Verification items for this drawing (mm, ordinates from the low corner). A direction names the side the tool comes from. Give positions to 0.01 mm unless a question says otherwise; leave off trailing zeros. Write each loop counter-clockwise with the first axis right and the second up, starting at its lowest first coordinate (ties: lowest second). Pieces come first, ordered by that corner, then holes. Notation, with made-up numbers: (8.25, -5.75) -> (47.25, -5.75) arc R28 ccw to (47.25, 30.25) -> close; hole circle Ø9 at (5, 45.5). An arc over 180 degrees is marked (long way). Answer as a JSON object with one key per item and string values.
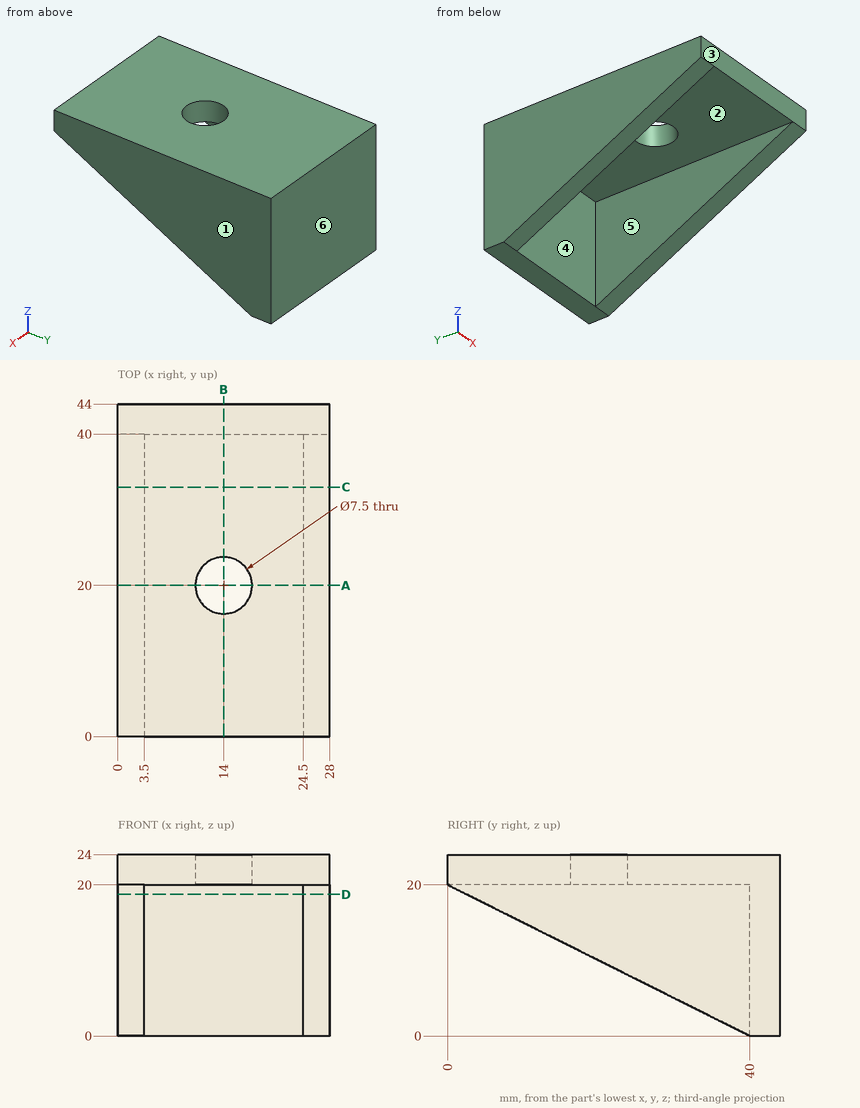
1. Sectioned sample at C-C, the plane y = 33. Enter the section's corners in (x, z), plus the area to 4 significant figures.
Determined:
{"outline": "(0, 3.5) -> (3.5, 3.5) -> (3.5, 20) -> (24.5, 20) -> (24.5, 3.5) -> (28, 3.5) -> (28, 24) -> (0, 24) -> close", "area": "227.5 mm^2"}
2. Scan lines: L1, parallel to Y at x = 14, z = 22.6; L2, parallel to X at y = 34, z = 13.5; L3, parallel to Z at x = 18.5, y = 37. Record each from-to range of solid material in increasing order. Write a range as [from, to].
Determined:
{"L1": "[0, 16.25], [23.75, 44]", "L2": "[0, 3.5], [24.5, 28]", "L3": "[20, 24]"}
3. Mould release check, pull along X, two halves, no side actions. Record for the marked faces 1, 2, 3 and 4: released by +X, released by -X, zero draft, split by the parting line, or undercut.
Determined:
{"face 1": "released by +X", "face 2": "undercut", "face 3": "zero draft", "face 4": "undercut"}
4. Sectioned sample at B-B, the plane x = 14. Enter the section's corners in (y, z), plus the area to 3 significant figures.
Determined:
{"outline": "(0, 20) -> (16.25, 20) -> (16.25, 24) -> (0, 24) -> close; (23.75, 20) -> (40, 20) -> (40, 0) -> (44, 0) -> (44, 24) -> (23.75, 24) -> close", "area": "226 mm^2"}
5. Go/stop test with flat-tipped pins: P1, Ø5, axis at x = 20, y = 21.5, coming from the -Z side; P2, Ø3, axis at y = 20.5, z = 8, coming from the +X side; P3, Ø10, axis at y = 18, z = 5.5, coming from the -X side; P4, Ø6, axis at x = 16, z = 8.5, coming from the -Y side. Record where each tip stops, or that it passes through.
Determined:
{"P1": "z = 20", "P2": "through", "P3": "x = 0", "P4": "y = 40"}
6. Sectioned sample at D-D, the plane z = 18.75. Enter the section's corners in (x, y).
Determined:
{"outline": "(0, 2.5) -> (3.5, 2.5) -> (3.5, 40) -> (24.5, 40) -> (24.5, 2.5) -> (28, 2.5) -> (28, 44) -> (0, 44) -> close"}
7. Access from +Z, -Z, +X, -X, +Y, -Y to the whole of each face (thin tool, end or side, straight path). Record for the marked faces 5 and 6.
Determined:
{"face 5": "-Z, -Y", "face 6": "+Z, -Z, +X, -X, +Y"}
8. Sectioned sample at A-A, the plane y = 20. Enter the section's corners in (x, z).
Determined:
{"outline": "(0, 10) -> (3.5, 10) -> (3.5, 20) -> (10.25, 20) -> (10.25, 24) -> (0, 24) -> close; (17.75, 20) -> (24.5, 20) -> (24.5, 10) -> (28, 10) -> (28, 24) -> (17.75, 24) -> close"}
